Design review of the part built by this model. Coordinates are the model's own, in mm. A direction names the side the tool comes from. Coordinates: 2 decimals unless noted, no trailing zeros. Write each loop counter-clockwise with the first axis right and the second up, starting at its lowest first coordinate (ties: lowest second). Pieces come first, ordered by that corner, then holes. Notation, with made-up numbers: (-26.75, -3) -> (-7.75, -3) arc R25 cw to (-7.75, 25) -> close; hole circle Ø4 at (-24.5, 82.5). An arc over 180 degrees is marked (long way). One line per question, with ' | ' between items. Start each with the question number.
Q1. Add section B-B on y = 10.5. State the section outline as (x, z) points (3 decimals), and give its area (3 significant figures).
Q2. Add section A-A on x = 5. State the section outline as (y, z) points (3 decimals).
Q3. For P1, Ø8, axis at x = 9, z = -9.5, coming from the -Y side; P2, Ø12, axis at x = 16, z = 4, coming from the +Y side; P3, Ø5, axis at x = 5.5, y = 44.5, coming from the +Z side (3 decimals); P4, Ø4, axis at x = 14.5, z = 6, coming from the +Y side, all flat-tipped, find the tip position at first contact; note any pin that passes through.
Q4. Wall thickness on probe 1 along X at (y, z) = (25.5, -9) (3 decimals); probe 2 along Z at (x, y) = (-7, 8) (3 decimals); probe 3 along Z at (x, y) = (21, 41.5) (3 decimals): over which ranges is each line inside the solid? List them lowest first.
Q5. Draft analysis for pull direction X (two halves, no side actions). For faces 3 (the flat face through (22.225, 25, 0)), 4 (the flat face through (0, 18, 12.7)), 5 (the flat face through (-25.4, 25, 0)), state which applies: pulls with the +X half, pulls with the -X half, needs draft (parallel to the pull), parting line crosses it, or undercut.
Q6. For faces 1 (the flat face through (0, 27, -9.525)), 2 (the flat face through (-1.763, 6.192, -10.407)), list the 3-axis set-ups (+Z, -Z, +X, -X, +Y, -Y) from which the entire face can be reached by the end or side of a thin tool; tool diameter is ignored.
Q7. Add section C-C on z = 7. State the section outline as (x, y) points (3 decimals).
Q8. Add section D-D on y = 40.5. State the section outline as (x, z) points (3 decimals).
from build123d import *

# Parameters (mm, degrees)
SKETCH1_W           = 50.8
SKETCH1_H           = 25.4
SKETCH1_W_2         = 44.45
SKETCH1_H_2         = 19.05
BOSS_EXTRUDE1_DEPTH = 50.8
CUT_EXTRUDE1_DEPTH  = 73.955945611
CUT_EXTRUDE2_DEPTH  = 73.955945611


with BuildPart() as part:
    # Sketch1 → Boss-Extrude1 (new body)
    with BuildSketch(Plane(origin=(0, 0, 0), x_dir=(1, 0, 0), z_dir=(0, 1, 0))):
        Rectangle(SKETCH1_W, SKETCH1_H)
        Rectangle(SKETCH1_W_2, SKETCH1_H_2, mode=Mode.SUBTRACT)
    extrude(amount=BOSS_EXTRUDE1_DEPTH)

    # Sketch2 → Cut-Extrude1 (cut, through all)
    with BuildSketch(Plane.ZY.offset(25.4)):
        Polygon((12.7, 50.8), (-12.7, 50.8), (12.7, 36.135303163), align=None)
    extrude(amount=-CUT_EXTRUDE1_DEPTH, mode=Mode.SUBTRACT)

    # Sketch3 → Cut-Extrude2 (cut, through all)
    with BuildSketch(Plane(origin=(25.4, 0, 0), x_dir=(0, 0, -1), z_dir=(1, 0, 0))):
        Polygon((12.7, 6.805909488), (-12.7, 0), (12.7, 0), align=None)
    extrude(amount=-CUT_EXTRUDE2_DEPTH, mode=Mode.SUBTRACT)


solid = part.part
Output values:
1) outline: (-25.4, -12.7) -> (25.4, -12.7) -> (25.4, 12.7) -> (-25.4, 12.7) -> close; hole (-22.225, -9.525) -> (22.225, -9.525) -> (22.225, 9.525) -> (-22.225, 9.525) -> close | area: 444 mm2
2) outline: (0, 12.7) -> (0.851, 9.525) -> (37.968, 9.525) -> (36.135, 12.7) -> close; (5.955, -9.525) -> (6.806, -12.7) -> (50.8, -12.7) -> (48.967, -9.525) -> close
3) P1: stops at y = 5.96 | P2: stops at y = 37.97 | P3: stops at z = -9.525 | P4: passes through
4) probe 1: x = -25.4 to -22.225, 22.225 to 25.4 | probe 2: z = -12.7 to -9.525, 9.525 to 12.7 | probe 3: z = -12.7 to -9.525
5) face 3: undercut | face 4: needs draft | face 5: pulls with the -X half
6) face 1: +Y, -Y | face 2: -Z, +X, -X, -Y
7) outline: (-25.4, 1.527) -> (-22.225, 1.527) -> (-22.225, 39.426) -> (-25.4, 39.426) -> close; (22.225, 1.527) -> (25.4, 1.527) -> (25.4, 39.426) -> (22.225, 39.426) -> close
8) outline: (-25.4, -12.7) -> (25.4, -12.7) -> (25.4, 5.14) -> (22.225, 5.14) -> (22.225, -9.525) -> (-22.225, -9.525) -> (-22.225, 5.14) -> (-25.4, 5.14) -> close
